Read the model definition and answer for the solid it produces. Units are mm, in the model's axes. Face numbers are marked on the shaded views. Give positions to 0.01 mm unless a question says otherwise; leave off trailing zeros. Order: outer loops, then holes, each group sorted by start corner. A loop starts at its lowest first (then second) coordinate and runs counter-clockwise, first axis right, second up.
Item 1: The mould has two halves that part along Z. Classify the marked faces 1, 2 and 3: +Z half, -Z half, draft (parallel to the pull), parting line (faces both ways), or undercut.
Item 2: A cutting plane is placed at B-B (x = -2.75). Write down the section's boundary in (y, z).
Item 3: Find the intervals of material crossed by line 1 along X through (y, z) = (2.25, -24.5); line 2 along Z through (x, y) = (-4, 9); line 3 along Z through (x, y) = (-2, 2), in increasing order.
Item 4: Given pin 1 Ø4 at (y, z) = (5.5, -31) entering from +X; pin 2 Ø6 at (y, z) = (5, -20.5) entering from +X; pin 3 Ø5 at (y, z) = (12.5, -23.5) entering from -X, each flat-ended and moving along its own axis, determine where each tip first touches the part or whether it passes through.
Item 5: A cutting plane is placed at A-A (y = 10.5). Write down the section's boundary in (x, z).
Item 6: A cutting plane is placed at C-C (z = -31.5). Write down the section's boundary in (x, y), plus the area to 3 significant figures.
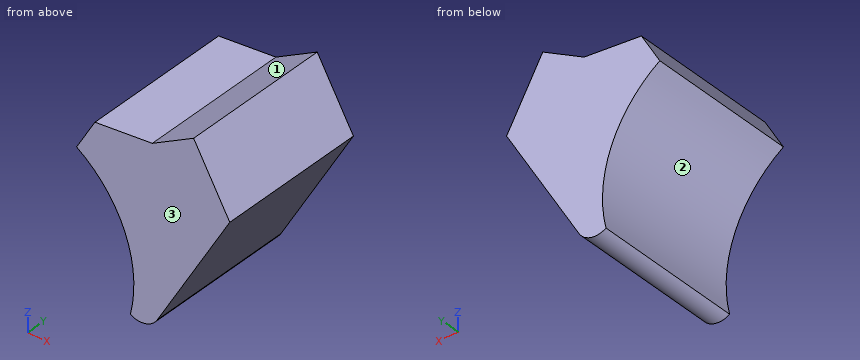
Autodesk Inventor part; units mm, degrees
ref_plane "YZ Plane" through (0, 0, 0) normal (1, 0, 0) x (0, 1, 0)
ref_plane "XZ Plane" through (0, 0, 0) normal (0, 1, 0) x (-1, 0, 0)
ref_plane "XY Plane" through (0, 0, 0) normal (0, 0, 1) x (1, 0, 0)
sketch "スケッチ2" plane through (0, 0, 0) normal (0, 1, 0) x (-1, 0, 0)
  line L0 (0, 0) -> (-8.6603, -15)
  line L1 (-8.6603, -15) -> (11.3397, -49.641)
  line L2 (73.7428, 0) -> (-22.3941, 0)
  line L3 (11.3397, -49.641) -> (5.9252, -52.7671) construction
  line L4 (0, 0) -> (-6.6711, 3.8516) construction
  line L5 (11.3397, -49.641) -> (24.3301, -42.141)
  line L6 (24.3301, -42.141) -> (0, 0)
  line L7 (0, 0) -> (8.2272, -4.75)
  line L8 (8.2272, -4.75) -> (-3.1754, -24.5)
  line L9 (-2.5935, -25.5079) -> (9.1002, -5.254)
  line L10 (9.1002, -5.254) -> (8.2272, -4.75)
  line L11 (-3.1754, -24.5) -> (2.5403, -27.8)
  line L12 (2.5403, -27.8) -> (12.2903, -10.9125)
  line L13 (12.2903, -10.9125) -> (6.5746, -7.6125)
  line L14 (6.5746, -7.6125) -> (-3.1754, -24.5)
  line L15 (11.3397, -49.641) -> (31.9282, -37.7543)
  line L16 (31.9282, -37.7543) -> (38.6416, -26.1264)
  line L17 (6.3397, -40.9808) -> (21.9282, -31.9808) construction
  line L18 (21.9282, -31.9808) -> (31.9282, -37.7543)
  line L19 (12.2903, -10.9125) -> (38.6416, -26.1264)
  line L20 (38.6416, -26.1264) -> (3.5066, -26.1264)
  line L21 (0, 0) -> (21.3397, 36.9615)
  line L22 (21.3397, 36.9615) -> (15.2136, 40.4985)
  line L23 (-0.5996, -1.0385) -> (60.009, -1.0385)
  circle A0 centre (21.3397, -13.5385) radius 12.5 construction
  circle A1 centre (21.3397, -13.5385) radius 10.5 construction
  circle A2 centre (20.5151, -34.5223) radius 10.5 construction
  circle A3 centre (20.5151, -34.5223) radius 11.5 construction
  circle A4 centre (20.5151, -34.5223) radius 12.5
  line L24 (8.3719, -37.4876) -> (11.3397, -49.641)
  line L25 (-2.3094, -23) -> (12.6388, -48.891)
  point P0 (9.2953, -16.1)
  point P1 (7.4475, -8.1165)
  point P2 (-2.3025, -25.004)
  point P3 (15.0841, -26.1264)
  point P4 (11.2545, -26.1264)
  point P5 (6.0668, -10.5079)
  point P6 (13.8325, -23.9586)
  point P7 (10.0702, -44.4421)
  point P8 (-1.7275, -24.0079)
  dimension "d34" = 25
  dimension "d11" = 60
  dimension "d12" = 60
  dimension "d13" = 40
  dimension "d15" = 15
  dimension "d16" = 9.5
  dimension "d17" = 1.0079
  dimension "d18" = 19.5
  dimension "d19" = 6.6
  dimension "d24" = 18
  dimension "d25" = 30
  dimension "d26" = 60
  dimension "d28" = 60
  dimension "d29" = 38
  dimension "d30" = 25
  dimension "d31" = 21
  dimension "d32" = 21
  dimension "d33" = 23
  dimension "d40" = 1.5
extrude "押し出し4" add sketch "スケッチ2" along normal blind 15 contours L6 L12 L11 L25 L9 | L6 A4 L20 L12 | L11 L12 L20 A4 L24 L25
fillet "フィレット1" radius 2 1 edges at (-10.0702, 7.5, -44.4421)
sketch "スケッチ3" plane through (0, 15, 0) normal (0, 1, 0) x (1, 0, 0)
  ellipse E0 centre (-16.5607, 22.817) end of major axis (-18.0607, 20.2189) minor radius 2.9999 (-18.4056, 20.4514) -> (-17.74, 20.0585) ccw
  ellipse E1 centre (-20.6882, 13.1623) end of major axis (-16.9382, 19.6575) minor radius 7.4997 (-13.3193, 14.5576) -> (-17.74, 20.0585) ccw
  line L0 (-13.3193, 14.5576) -> (-11.4591, 4.7323)
  line L1 (-11.4591, 4.7323) -> (-7.1359, 7.9366)
  line L2 (-7.1359, 7.9366) -> (-2.1359, 16.5968)
  line L3 (-2.1359, 16.5968) -> (-6.4659, 19.0967)
  line L4 (-6.4659, 19.0967) -> (-18.4056, 20.4514)
  line L5 (-6.0668, 10.5079) -> (1.7275, 24.0079)
  line L6 (-1.9475, 17.6428) -> (-6.1462, 20.0669)
  line L7 (-6.1462, 20.0669) -> (-11.9669, 20.7273)
  line L8 (-13.8325, 23.9586) -> (-6.0668, 10.5079)
  point P0 (0, 0)
  point P1 (2.5935, 25.5079)
  dimension "d36" = 1
  dimension "d37" = 1
extrude "押し出し5" cut sketch "スケッチ3" against normal through all contours L8 L7 L6 L5 L3 L4 | L4 L3 L5 L8
equation "\"d37\" = d36"
properties part number "base_backwall_setter_under"
Response values:
1. face 1: +Z half
1. face 2: undercut
1. face 3: draft
2. outline: (0, -31.76) - (15, -31.76) - (15, -18.11) - (0, -18.11) - close
3. line 1: x = -13.04 to 1.44
3. line 2: z = -33.93 to -18.83
3. line 3: z = -30.46 to -17.67
4. pin 1: stops at x = -1.15
4. pin 2: stops at x = 1.43
4. pin 3: stops at x = -13.83
5. outline: (-13.83, -23.96) arc R12.5 cw to (-8.37, -37.49) arc R2 ccw to (-5.63, -36.76) - (1.73, -24.01) - (-1.95, -17.64) - (-6.15, -20.07) - (-11.97, -20.73) - close
6. outline: (-8.39, 0) - (-2.6, 0) - (-2.6, 15) - (-8.39, 15) - close
6. area: 86.8 mm2
